Could you check a few things on this drawing? It's one solid part, dimensions in mm from its lowest x, y, z. Give positions to 0.01 mm unless a question says otherwise; leave off trailing zeros. Order: outer loops, then holes, each group sorted by start corner. A loop starts at its lowest first (then second) coordinate and runs counter-clockwise, first axis right, second up.
Item 1: I'm going to push a flat-ended pin straight in: pin 1 Ø4 at (x, z) = (55.88, 19) entering from -Y. Where does the tip first touch, or does it pass through?
Item 2: I want a section at B-B, the plane z = 32.5. Write out the boundary of the cut face in (x, y).
Item 3: If I drill on line 1 along Z through (x, y) = (32.5, 0.6); line 2 along X through (y, z) = (0.5, 19); line 3 along X through (y, z) = (0.75, 59.5), over which ranges is the centre line in solid material (lowest first)?
Item 4: I want a section at C-C, the plane y = 0.6. Write out the boundary of the cut face in (x, z), then the cut area to 3 significant figures.
Item 5: I want a section at A-A, the plane x = 32.5. Write out the boundary of the cut face in (y, z).
Item 6: I want a section at D-D, the plane z = 19. Write out the boundary of the cut face in (x, y).
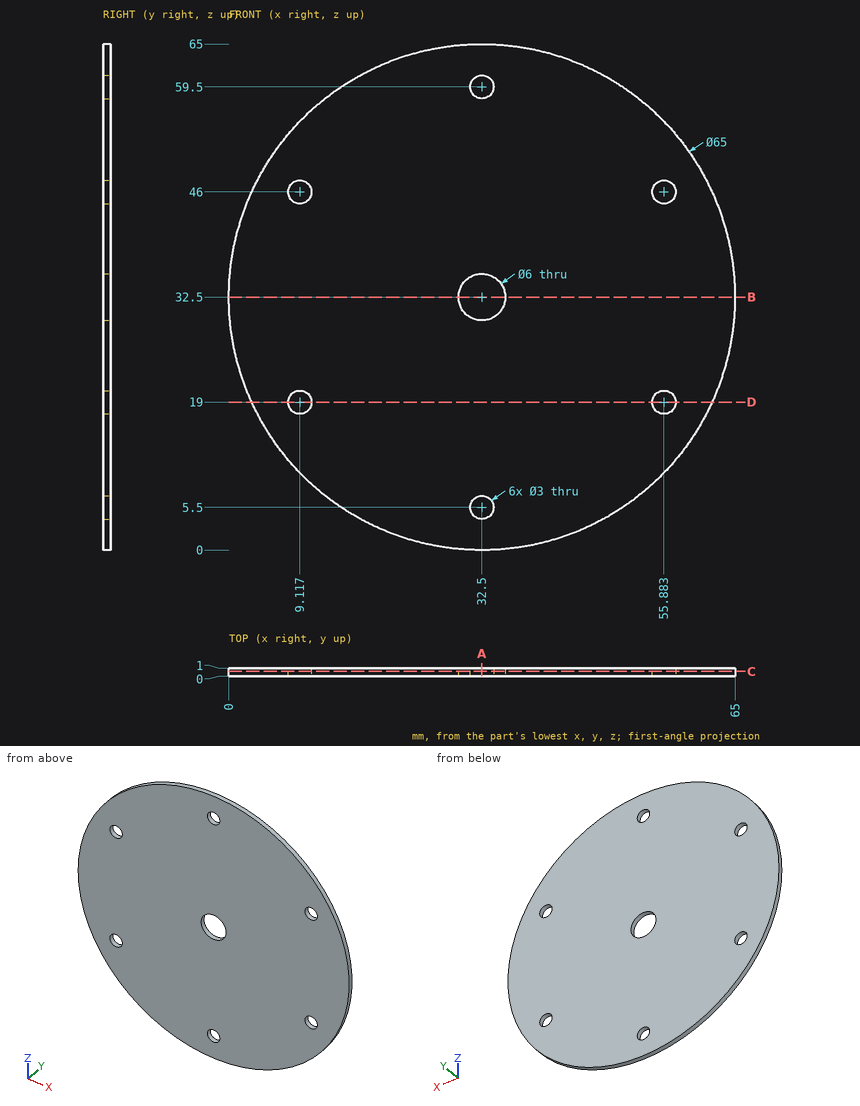
Results list:
1. pin 1: stops at y = 0
2. outline: (0, 0) - (29.5, 0) - (29.5, 1) - (0, 1) - close; (35.5, 0) - (65, 0) - (65, 1) - (35.5, 1) - close
3. line 1: z = 0 to 4, 7 to 29.5, 35.5 to 58, 61 to 65
3. line 2: x = 2.94 to 7.62, 10.62 to 54.38, 57.38 to 62.06
3. line 3: x = 14.41 to 31, 34 to 50.59
4. outline: circle Ø65 at (32.5, 32.5); hole circle Ø3 at (9.12, 19); hole circle Ø3 at (9.12, 46); hole circle Ø6 at (32.5, 32.5); hole circle Ø3 at (32.5, 5.5); hole circle Ø3 at (32.5, 59.5); hole circle Ø3 at (55.88, 19); hole circle Ø3 at (55.88, 46)
4. area: 3,250 mm2
5. outline: (0, 0) - (1, 0) - (1, 4) - (0, 4) - close; (0, 7) - (1, 7) - (1, 29.5) - (0, 29.5) - close; (0, 35.5) - (1, 35.5) - (1, 58) - (0, 58) - close; (0, 61) - (1, 61) - (1, 65) - (0, 65) - close
6. outline: (2.94, 0) - (7.62, 0) - (7.62, 1) - (2.94, 1) - close; (10.62, 0) - (54.38, 0) - (54.38, 1) - (10.62, 1) - close; (57.38, 0) - (62.06, 0) - (62.06, 1) - (57.38, 1) - close
